Geometry: final body of the model. Coordinates: model frame, mm. A direction names the side the tool comes from. Round coordinates to 2 decimals unless told otherwise and drop trailing zeros. Order: outer loops, then holes, each group sorted by start corner. A loop starts at its lowest first (then second) coordinate and runs counter-clockwise, first axis right, second up. Notation, with made-up numbers: M -28,16.25 L 3,16.25 A27 cw 3,49.25 Z; hole C 20.25,-27.75 d10. An arc over 180 degrees is marked long. Return JSON: item names as keys, results as strings. Group by question number.
Q1. Cut plane C-C on y = 5. Output: boundary loops of the cut face in (x, z), and give its area (3 significant figures).
Q2. Cut plane D-D on x = 5.5. Output: boundary loops of the cut face in (y, z).
Q3. Access query for faces 5 (the face through (21, -13, 3)), 6 (the face through (-16, -6, 3)), 7 (the face through (11.18, 4.63, 4.46)). Directions: +Z, -Z, +X, -X, +Y, -Y. A direction counts if a zero-diameter tool reaches every point of the face in a straight line with its end or side. Return the directions, or none.
Q4. Contact query for flat-ended pins moving along their axis: pin 1 (2 mm diameter, centred on x = 24, z = 4, fed in from +Y); pin 2 (14.5 mm diameter, centred on x = 0, y = 0, fed in from -Z); pin 3 (2 mm diameter, centred on y = -4.5, z = 5, fed in from -X); pin 4 (8 mm diameter, centred on x = -2.5, y = 9, fed in from -Z). Output: stop coordinate, or through.
Q5. Cut plane B-B on x = -23. Output: boundary loops of the cut face in (y, z).
Q6. Mould query, pull axis X, two halves, no side actions, for faces 1 (the face through (2, 9, 2)), 2 (the face through (-21.474, -15.218, 3.019)), 3 (the face through (-16.301, -12.715, 3.549)), 4 (the face through (-21, -13, 3)). Classes: released by +X, released by -X, zero draft, split by the parting line, or undercut.
Q7. Ray query, probe 1 along X at (y, z) = (-16, 3.5); probe 2 along Y at (x, z) = (0, 3.8); probe 3 along Y at (x, z) = (0, 0.7). Return the intervals inside material, ascending.
Q8. Cut plane A-A on z = 3.5. Count the separate pieces of the cut face and the enclosed holes in it, and give its area (3 significant figures).
Autodesk Inventor part; units mm, degrees
ref_plane "YZ Plane" through (0, 0, 0) normal (1, 0, 0) x (0, 1, 0)
ref_plane "XZ Plane" through (0, 0, 0) normal (0, 1, 0) x (-1, 0, 0)
ref_plane "XY Plane" through (0, 0, 0) normal (0, 0, 1) x (1, 0, 0)
sketch "Skizze1" plane through (0, 0, 0) normal (0, 0, 1) x (1, 0, 0)
  line L0 (0, 22.4) -> (0, -22.4)
  line L1 (-22.4, 0) -> (22.4, 0)
  line L2 (-16, 16) -> (16, 16)
  line L3 (16, 16) -> (16, -16)
  line L4 (16, -16) -> (-16, -16)
  line L5 (-16, -16) -> (-16, 16)
  circle A0 centre (0, 0) radius 12.1
  dimension "d0" = 32
  dimension "d1" = 32
  dimension "d2" = 24.2
extrude "Extrusion1" add sketch "Skizze1" along normal blind 7 contours L2 L3 L1 A0 L0 | L0 A0 L1 L5 L2 | L1 L3 L4 L0 A0 | A0 L0 L4 L5 L1
sketch "Skizze2" plane through (16, -16, 0) normal (1, 0, 0) x (0, 0, -1)
  line L0 (-7, 32) -> (-7, 0)
  line L1 (0, 32) -> (0, 0)
  line L2 (-7, 0) -> (0, 0)
  line L3 (0, 0) -> (0, 3)
  line L4 (0, 3) -> (-7, 3)
  line L5 (-7, 3) -> (-7, 0)
  point P0 (0, 16)
  point P1 (-7, 3)
  dimension "d5" = 3
sketch "Skizze3" plane through (-16, -16, 0) normal (-1, 0, 0) x (0, 0, 1)
  line L0 (7, 32) -> (7, 0)
  line L1 (0, 32) -> (0, 0)
  line L2 (7, 0) -> (0, 0)
  line L3 (0, 0) -> (0, 3)
  line L4 (0, 3) -> (7, 3)
  line L5 (7, 3) -> (7, 0)
  point P0 (0, 16)
  point P1 (7, 3)
  dimension "d6" = 3
extrude "Extrusion2" add sketch "Skizze3" along normal blind 10.5
extrude "Extrusion3" add sketch "Skizze2" along normal blind 10.5
sketch "Skizze4" plane through (0, 0, 0) normal (0, 0, -1) x (-1, 0, 0)
  circle A0 centre (0, 0) radius 12.1
  circle A1 centre (0, 0) radius 12.1
  circle A2 centre (0, 0) radius 9
  dimension "d11" = 24.2
  dimension "d12" = 18
extrude "Extrusion4" add sketch "Skizze4" against normal blind 2
fillet "Rundung1" radius 16 2 edges at (16, 16, 3.5) (-16, 16, 3.5)
sketch "Skizze5" plane through (16, -13, 7) normal (0, 1, 0) x (1, 0, 0)
  circle A0 centre (-39, 3.5) radius 1.6
  line L0 (-32, 7) -> (-42.5, 7)
  line L1 (-42.5, 0) -> (-42.5, 7)
  circle A1 centre (7, 3.5) radius 1.6
  line L2 (0, 7) -> (10.5, 7)
  line L3 (10.5, 7) -> (10.5, 0)
  point P0 (-16, 7)
  dimension "d16" = 3.2
  dimension "d17" = 3.5
  dimension "d18" = 3.5
  dimension "d19" = 3.2
  dimension "d20" = 3.5
  dimension "d21" = 3.5
extrude "Extrusion5" cut sketch "Skizze5" against normal up to surface (3 mm away)
fillet "Rundung2" radius 1 2 edges at (-16, -13, 3.5) (16, -13, 3.5)
sketch "Skizze6" plane through (-26.5, -16, 0) normal (0, -1, 0) x (1, 0, 0)
  line L0 (0, 0) -> (0, 7)
  line L1 (53, 7) -> (53, 0)
  line L2 (0, 7) -> (53, 7)
  line L3 (53, 7) -> (53, 0)
  line L4 (53, 0) -> (0, 0)
  line L5 (0, 0) -> (0, 7)
  circle A0 centre (3.5, 3.5) radius 1.6
  circle A1 centre (3.5, 3.5) radius 1.6
  circle A2 centre (49.5, 3.5) radius 1.6
  circle A3 centre (49.5, 3.5) radius 1.6
  point P0 (26.5, 0)
  dimension "d25" = 3.2
  dimension "d26" = 3.2
extrude "Extrusion6" add sketch "Skizze6" along normal blind 1.5
properties part number "_3D-Druck"
Result sheet:
{
 "1": {"outline": "M -15.2,0 L -7.48,0 L -7.48,2 L -11.02,2 L -11.02,7 L -15.2,7 Z; M 7.48,0 L 15.2,0 L 15.2,7 L 11.02,7 L 11.02,2 L 7.48,2 Z", "area": "72.7 mm²"},
 "2": {"outline": "M -17.5,0 L -7.12,0 L -7.12,2 L -10.78,2 L -10.78,7 L -17.5,7 Z; M 7.12,0 L 15.03,0 L 15.03,7 L 10.78,7 L 10.78,2 L 7.12,2 Z"},
 "3": {"face 5": "+Z, -Z, +X, +Y", "face 6": "+Z, -Z, -X, +Y", "face 7": "+Z"},
 "4": {"pin 1": "stops at y = -13", "pin 2": "passes through", "pin 3": "stops at x = -16", "pin 4": "stops at z = 0"},
 "5": {"outline": "M -17.5,0 L -13,0 L -13,1.9 L -17.5,1.9 Z; M -17.5,5.1 L -13,5.1 L -13,7 L -17.5,7 Z"},
 "6": {"face 1": "undercut", "face 2": "undercut", "face 3": "released by -X", "face 4": "zero draft"},
 "7": {"probe 1": "x = -26.5 to -24.6, -21.4 to 21.4, 24.6 to 26.5", "probe 2": "y = -17.5 to -12.1, 12.1 to 16", "probe 3": "y = -17.5 to -9, 9 to 16"},
 "8": {"separate pieces": "3", "enclosed holes": "1", "area": "568 mm²"}
}
